Check sheet for the modelled part. Datum: model origin and axes. Units: mm. A direction names the side the tool comes from. Give positions to 0.01 mm unless a question says otherwise; leave off trailing zeros. Order: outer loops, then holes, each group sorted by start corner. A loop starts at its lowest first (then second) coordinate and runs counter-clockwise, first axis right, second up. Notation, with made-up numbers: (52.25, -9.5) -> (111.25, -9.5) arc R29 cw to (111.25, 28.5) -> close; hole circle Ø11 at (89.25, 0). An arc over 180 degrees is marked (long way). One line per question, with ' | ' between items.
Autodesk Inventor part; units mm, degrees
ref_plane "YZ Plane" through (0, 0, 0) normal (1, 0, 0) x (0, 1, 0)
ref_plane "XZ Plane" through (0, 0, 0) normal (0, 1, 0) x (-1, 0, 0)
ref_plane "XY Plane" through (0, 0, 0) normal (0, 0, 1) x (1, 0, 0)
sketch "Sketch1" plane through (0, 0, 0) normal (0, 0, 1) x (1, 0, 0)
  line L0 (-17.78, 0) -> (17.78, 0)
  line L1 (0, -17.78) -> (0, 17.78)
  line L2 (-12.7, 12.7) -> (12.7, 12.7)
  line L3 (12.7, 12.7) -> (12.7, -12.7)
  line L4 (12.7, -12.7) -> (-12.7, -12.7)
  line L5 (-12.7, -12.7) -> (-12.7, 12.7)
  line L6 (9.525, 9.525) -> (-9.525, 9.525)
  line L7 (-9.525, 9.525) -> (-9.525, -9.525)
  line L8 (-9.525, -9.525) -> (9.525, -9.525)
  line L9 (9.525, -9.525) -> (9.525, 9.525)
  point P0 (0, 0)
  point P1 (-12.7, 0)
  point P2 (0, 12.7)
  dimension "d0" = 25.4
  dimension "d1" = 3.175
extrude "Extrusion1" add sketch "Sketch1" along normal mid plane 406.4 contours L5 L2 L1 L6 L7 L0 | L0 L7 L8 L1 L4 L5 | L1 L8 L9 L0 L3 L4 | L2 L3 L0 L9 L6 L1
sketch "Sketch3" plane through (-12.7, 12.7, 203.2) normal (0, 1, 0) x (1, 0, 0)
  line L0 (0, 0) -> (25.4, 0)
  line L1 (25.4, 0) -> (25.4, 406.4)
  line L2 (25.4, 406.4) -> (0, 406.4)
  line L3 (0, 406.4) -> (0, 0)
  line L4 (0, 203.2) -> (25.4, 203.2) construction
  line L5 (0, 0) -> (25.4, 14.6647)
  line L6 (0, 406.4) -> (25.4, 391.7353)
  line L7 (0, 406.4) -> (25.4, 406.4)
  line L8 (25.4, 391.7353) -> (25.4, 406.4)
  point P0 (12.7, 203.2)
  dimension "d7" = 30
extrude "Extrusion3" cut sketch "Sketch3" against normal through all contours L5 L1 L0
sketch "Sketch4" plane through (-12.7, 12.7, -203.2) normal (0, 1, 0) x (1, 0, 0)
  line L0 (25.4, -391.7353) -> (25.4, 0)
  line L1 (25.4, 0) -> (0, 0)
  line L2 (0, 0) -> (25.4, -43.9941)
  point P0 (12.7, -203.2)
  dimension "d10" = 60
extrude "Extrusion4" cut sketch "Sketch4" against normal through all
properties part number "tubing_template_0.125" material "Aluminum-6061"
Q1. Thickness scan on line 1 (X direction, y = 9.25, z = 112.5) (3 decimals); line 2 (Z direction, x = 10.5, y = -5). Record the ranges inside material, lowest first.
Result sheet:
line 1: x = -12.7 to -9.525, 9.525 to 12.7 | line 2: z = -163.02 to 189.81
Q2. Access from +Z, -Z, +X, -X, +Y, -Y to the whole of each face (thin tool, end or side, straight path). Record for faces 1 (the face through (0, 9.525, -1)), 2 (the face through (-0.18, -11.11, 195.97)).
Result sheet:
face 1: +Z, -Z | face 2: +Z, +X, +Y, -Y
Q3. Depth check by flat-ended pin: pin 1 Ø2 at (x, y) = (-9, -6) entering from -Z. Enter the tip coordinate at first touch or a pass-through.
Result sheet:
pin 1: stops at z = -198.52
Q4. Section check C-C (x = 5.5). Enter the section's corners in (y, z) (3 decimals).
Result sheet:
outline: (-12.7, -171.677) -> (-9.525, -171.677) -> (-9.525, 192.692) -> (-12.7, 192.692) -> close; (9.525, -171.677) -> (12.7, -171.677) -> (12.7, 192.692) -> (9.525, 192.692) -> close
Q5. Section check B-B (z = 150.5). Enter the section's corners in (x, y) (3 decimals), and give its area (3 significant figures).
Result sheet:
outline: (-12.7, -12.7) -> (12.7, -12.7) -> (12.7, 12.7) -> (-12.7, 12.7) -> close; hole (-9.525, -9.525) -> (9.525, -9.525) -> (9.525, 9.525) -> (-9.525, 9.525) -> close | area: 282 mm2
Q6. Section check D-D (z = -168.5). Enter the section's corners in (x, y) (3 decimals).
Result sheet:
outline: (-12.7, -12.7) -> (7.334, -12.7) -> (7.334, -9.525) -> (-9.525, -9.525) -> (-9.525, 9.525) -> (7.334, 9.525) -> (7.334, 12.7) -> (-12.7, 12.7) -> close
Q7. Mould release check, pull along Y, two halves, no side actions. Record for faces 3 (the face through (0, 12.7, -3)), 4 (the face through (9.525, 0, 10)), 5 (the face through (12.7, 0, 12)), 6 (the face through (0, -12.7, -3)): pulls with the +Y half, pulls with the -Y half, needs draft (parallel to the pull), parting line crosses it, or undercut.
Result sheet:
face 3: pulls with the +Y half | face 4: undercut | face 5: needs draft | face 6: pulls with the -Y half
Q8. Section check A-A (y = -3.5). Enter the section's corners in (x, z) (3 decimals), and give its area (3 significant figures).
Result sheet:
outline: (-12.7, -203.2) -> (-9.525, -197.701) -> (-9.525, 201.367) -> (-12.7, 203.2) -> close; (9.525, -164.705) -> (12.7, -159.206) -> (12.7, 188.535) -> (9.525, 190.368) -> close | area: 2,390 mm2
